Here's how the part is built. I have some questions about the finished solid (model axes, mm). Round coordinates to 2 decimals unless told otherwise and drop trailing zeros. Loops run counter-clockwise (first coordinate to the right, second up) from the corner with the lowest first, then second, coordinate; pieces in that order, holes last. Notation, with made-up numbers: M 62,-4.5 L 116,-4.5 A13 cw 116,7.5 Z; hole C 62.25,82 d3. An arc over 180 degrees is marked long. Use a Markdown table: item, result.
from build123d import *

# Parameters (mm, degrees)
F0_R     = 9.525
F1_DEPTH = 15.875


with BuildPart() as f1:
    # F0 (on Front) → F1 (new body, symmetric)
    with BuildSketch(Plane.XZ):
        with BuildLine():
            ThreePointArc((-300.0802086054, 0.9095984296), (-302.3966793747, 0.2294727468), (-304.8, 0))
            ThreePointArc((-304.8, 0), (-159.858648812, -71.8136278274), (0, -96.52))
            Line((0, -96.52), (0, -93.0700078607))
            ThreePointArc((0, -93.0700078607), (-157.2261889724, -69.0256273648), (-300.0802086054, 0.9095984296))
        make_face()
        with BuildLine():
            ThreePointArc((-292.1, 12.7), (-313.7802561211, 21.6802561211), (-304.8, 0))
            ThreePointArc((-304.8, 0), (-302.3966793747, 0.2294727468), (-300.0802086054, 0.9095984296))
            ThreePointArc((-300.0802086054, 0.9095984296), (-294.2826013028, 5.5814099258), (-292.1, 12.7))
        make_face()
        with Locations((-304.8, 12.7)):
            Circle(F0_R, mode=Mode.SUBTRACT)
        with BuildLine():
            Line((0, -93.0700078607), (0, -96.52))
            ThreePointArc((0, -96.52), (159.858648812, -71.8136278274), (304.8, 0))
            ThreePointArc((304.8, 0), (302.3966793747, 0.2294727468), (300.0802086054, 0.9095984296))
            ThreePointArc((300.0802086054, 0.9095984296), (157.2261889724, -69.0256273648), (0, -93.0700078607))
        make_face()
        with BuildLine():
            ThreePointArc((300.0802086054, 0.9095984296), (302.3966793747, 0.2294727468), (304.8, 0))
            ThreePointArc((304.8, 0), (313.7802561211, 3.7197438789), (317.5, 12.7))
            ThreePointArc((317.5, 12.7), (297.6814099258, 23.2173986972), (300.0802086054, 0.9095984296))
        make_face()
        with Locations((304.8, 12.7)):
            Circle(F0_R, mode=Mode.SUBTRACT)
    extrude(amount=F1_DEPTH, both=True)


solid = f1.part
1. For pin 1 Ø5 at (x, y) = (129.5, -12) entering from -Z; pin 2 Ø8 at (y, z) = (-4, -51) entering from -X; pin 3 Ø1 at (x, y) = (-59.5, 4.5) entering from -Z, each with a flat end and sliding along its axis, tell me the tip position at first contact or that it passes through.
Answer sheet:
| item | result |
|---|---|
| pin 1 | z = -81.06 |
| pin 2 | x = -223.59 |
| pin 3 | z = -93.22 |
2. Imagine slicing it at A-A, the plane y = -3. Write out the boundary of the cut face in (x, z) (3 decimals), then the cut area to 3 significant figures.
Answer sheet:
| item | result |
|---|---|
| outline | M -304.8,0 A529.523 ccw 304.8,0 A12.7 ccw long 300.08,0.91 A526.073 cw -300.08,0.91 A12.7 ccw long Z; hole C -304.8,12.7 d19.05; hole C 304.8,12.7 d19.05 |
| area | 2,660 mm2 |
3. I need wall thicknesses on probe 1 along X at (y, z) = (4, 12); probe 2 along X at (y, z) = (8.5, 15); probe 3 along Z at (x, y) = (304, -4). Which ranges of each line are inside material? Lowest first, please. Write a range as from..to.
Answer sheet:
| item | result |
|---|---|
| probe 1 | -317.48..-314.3, -295.3..-292.12, 292.12..295.3, 314.3..317.48 |
| probe 2 | -317.29..-314.04, -295.56..-292.31, 292.31..295.56, 314.04..317.29 |
| probe 3 | -0.56..3.21, 22.19..25.37 |
4. We'd pull the mould along X, two halves only. Please class faces 1 (the face through (-4.5, -0.2, -96.5)), 2 (the face through (4.47, -0.22, -93.05)), 3 (the face through (-25, 15.875, -94)): +X half, -X half, draft (parallel to the pull), parting line (faces both ways), or undercut.
Answer sheet:
| item | result |
|---|---|
| face 1 | parting line |
| face 2 | undercut |
| face 3 | draft |
